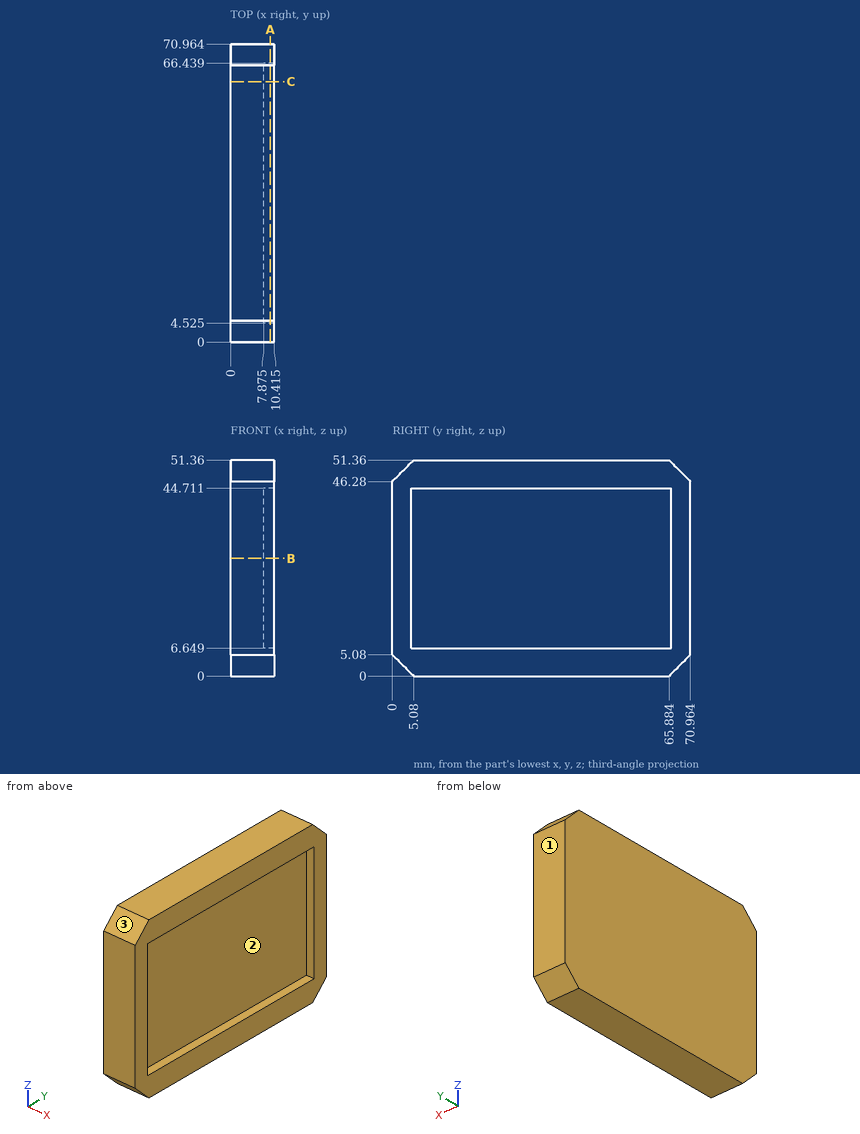
For this review, use the dimensioned drawing (mm, ordinates from the lowest corner) and the shaded views. Coordinates: 2 decimals unless noted, no trailing zeros. Loops run counter-clockwise (first coordinate to the right, second up) from the corner with the lowest first, then second, coordinate; pieces in that order, holes last. Notation, with made-up numbers: (43, 71.25) - (64, 71.25) arc R24 ccw to (64, 81.25) - close; hole circle Ø6 at (6, 70.5). An arc over 180 degrees is marked (long way). Use one line per item in the form item = value. Start each with the question number.
1) Draft analysis for pull direction Y (two halves, no side actions). For the marked faces 1, 2 and 3, state which applies: released by +Y, released by -Y, zero draft, split by the parting line, or undercut.
2) To check wall thickness, follow probe 1 along Y at (x, z) = (9.5, 30) (1 decimal); probe 2 along Z at (x, y) = (9.75, 45); probe 3 along X at (y, z) = (40, 40) (1 decimal). State the ranges of each line that lie inside material, in increasing order. Write a range as from..to.
3) Take a section at A-A (x = 9.5). State the section outline as (y, z) points (1 decimal).
4) For pin 1 (5 mm diameter, centred on y = 28.5, z = 17, fed in from +X) (1 decimal), flat-tipped, find the tip position at first contact; note if it passes through.
5) Take a section at B-B (z = 28). State the section outline as (x, y) points (1 decimal), plus the area to 3 significant figures.
6) Take a section at C-C (y = 62). State the section outline as (x, z) points (1 decimal), plus the area to 3 significant figures.
From the geometry:
q1.face_1 = released by +Y
q1.face_2 = undercut
q1.face_3 = released by -Y
q2.probe_1 = 0..4.5, 66.4..71
q2.probe_2 = 0..6.65, 44.71..51.36
q2.probe_3 = 0..7.9
q3.outline = (0, 5.1) - (5.1, 0) - (65.9, 0) - (71, 5.1) - (71, 46.3) - (65.9, 51.4) - (5.1, 51.4) - (0, 46.3) - close; hole (4.5, 6.6) - (66.4, 6.6) - (66.4, 44.7) - (4.5, 44.7) - close
q4.pin_1 = 7.9
q5.outline = (0, 0) - (10.4, 0) - (10.4, 4.5) - (7.9, 4.5) - (7.9, 66.4) - (10.4, 66.4) - (10.4, 71) - (0, 71) - close
q5.area = 582 mm2
q6.outline = (0, 0) - (10.4, 0) - (10.4, 6.6) - (7.9, 6.6) - (7.9, 44.7) - (10.4, 44.7) - (10.4, 51.4) - (0, 51.4) - close
q6.area = 438 mm2
